Here's how the part is built. I have some questions about the finished solid (model axes, mm). A direction names the side the tool comes from. Round coordinates to 2 decimals unless told otherwise and drop trailing zeros. Order: outer loops, then holes, each group sorted by start corner. A loop starts at its lowest first (then second) coordinate and runs counter-clockwise, first axis right, second up. Notation, with made-up numbers: (54, 84.25) - (66, 84.25) arc R25 ccw to (66, 112.25) - close; hole circle Ø1 at (82.25, 30.25). An arc over 180 degrees is marked (long way). Answer as a JSON object with one key per item and string values.
Autodesk Inventor part; units mm, degrees
ref_plane "YZ Plane" through (0, 0, 0) normal (1, 0, 0) x (0, 1, 0)
ref_plane "XZ Plane" through (0, 0, 0) normal (0, 1, 0) x (-1, 0, 0)
ref_plane "XY Plane" through (0, 0, 0) normal (0, 0, 1) x (1, 0, 0)
sketch "Sketch1" plane through (0, 0, 0) normal (0, 1, 0) x (-1, 0, 0)
  circle A0 centre (0, 0) radius 2.1
  circle A1 centre (0, 0) radius 4
  circle A2 centre (0, 0) radius 5
  dimension "d0" = 4.2
  dimension "d1" = 8
  dimension "d2" = 10
extrude "Extrusion1" add sketch "Sketch1" along normal blind 8 contours A1
extrude "Extrusion2" add sketch "Sketch1" along normal blind 0.5
thread "Thread1"
properties part number "Návarek M5" material "Aluminum 6061"
1. For faces 1 (the face through (0.867, 4.198, 3.905)), 2 (the face through (-2, 8, -2)), which set-ups out of +Z, -Z, +X, -X, +Y, -Y let a thin tool reach every point of the face, with its end or its side?
Responses:
{"face 1": "+Y", "face 2": "+Z, -Z, +X, -X, +Y"}
2. Imagine slicing it at A-A (z = 0). List the corners of the cut face in (x, y) for me, plus the area to 3 significant figures.
Responses:
{"outline": "(-5, 0) - (5, 0) - (5, 0.5) - (4, 0.5) - (4, 8) - (2.1, 8) - (2.1, 0.5) - (-2.1, 0.5) - (-2.1, 8) - (-4, 8) - (-4, 0.5) - (-5, 0.5) - close", "area": "33.5 mm2"}
3. Imagine slicing it at D-D (x = -3). List the corners of the cut face in (y, z) for me, plus the area to 3 significant figures.
Responses:
{"outline": "(0, -4) - (0.5, -4) - (0.5, -2.65) - (8, -2.65) - (8, 2.65) - (0.5, 2.65) - (0.5, 4) - (0, 4) - close", "area": "43.7 mm2"}
4. If I drill on L1, parallel to Z at x = 0, y = 5.5; L2, parallel to Y at x = -2, z = -4.25; L3, parallel to X at y = 4.5, z = 1, over which ranges is the centre line in solid material (lowest first)? Write a range as [from, to].
Responses:
{"L1": "[-4, -2.1], [2.1, 4]", "L2": "[0, 0.5]", "L3": "[-3.87, -1.85], [1.85, 3.87]"}
5. For P1, Ø2, axis at x = 3, z = 1.5, coming from the -Y side; P2, Ø2, axis at x = -0.5, z = 0.5, coming from the +Y side; P3, Ø3, axis at x = 0, y = 4.5, coming from the +Z side; P4, Ø1, axis at y = 3.5, z = 2.5, coming from the +X side, each with a flat end and sliding along its axis, tell me the tip position at first contact or that it passes through.
Responses:
{"P1": "y = 0", "P2": "y = 0.5", "P3": "z = 4", "P4": "x = 3.46"}
6. Thinking about a two-plate mould opening in X: for faces 3 (the face through (0, 0, 0)), 4 (the face through (0, 0.5, 0)), 5 (the face through (1.08, 0.25, 4.88)), 6 (the face through (-2.003, 4.198, -0.631)), which applies, pulls with the +X half, pulls with the -X half, needs draft (parallel to the pull), parting line crosses it, or undercut?
Responses:
{"face 3": "needs draft", "face 4": "undercut", "face 5": "parting line crosses it", "face 6": "undercut"}
7. Imagine slicing it at C-C (y = 2.25). List the corners of the cut face in (x, z) for me, plus the area to 3 significant figures.
Responses:
{"outline": "circle Ø8 at (0, 0); hole circle Ø4.2 at (0, 0)", "area": "36.4 mm2"}
8. Imagine slicing it at B-B (x = 0). List the corners of the cut face in (y, z) for me, plus the area to 3 significant figures.
Responses:
{"outline": "(0, -5) - (0.5, -5) - (0.5, -4) - (8, -4) - (8, -2.1) - (0.5, -2.1) - (0.5, 2.1) - (8, 2.1) - (8, 4) - (0.5, 4) - (0.5, 5) - (0, 5) - close", "area": "33.5 mm2"}
